Job drawing, mm, ordinate dimensions from the low corner. One solid piece. Round coordinates to 2 decimals unless told otherwise and drop trailing zeros. Loops run counter-clockwise (first coordinate to the right, second up) from the corner with the lowest first, then second, coordinate; pieces in that order, holes last.
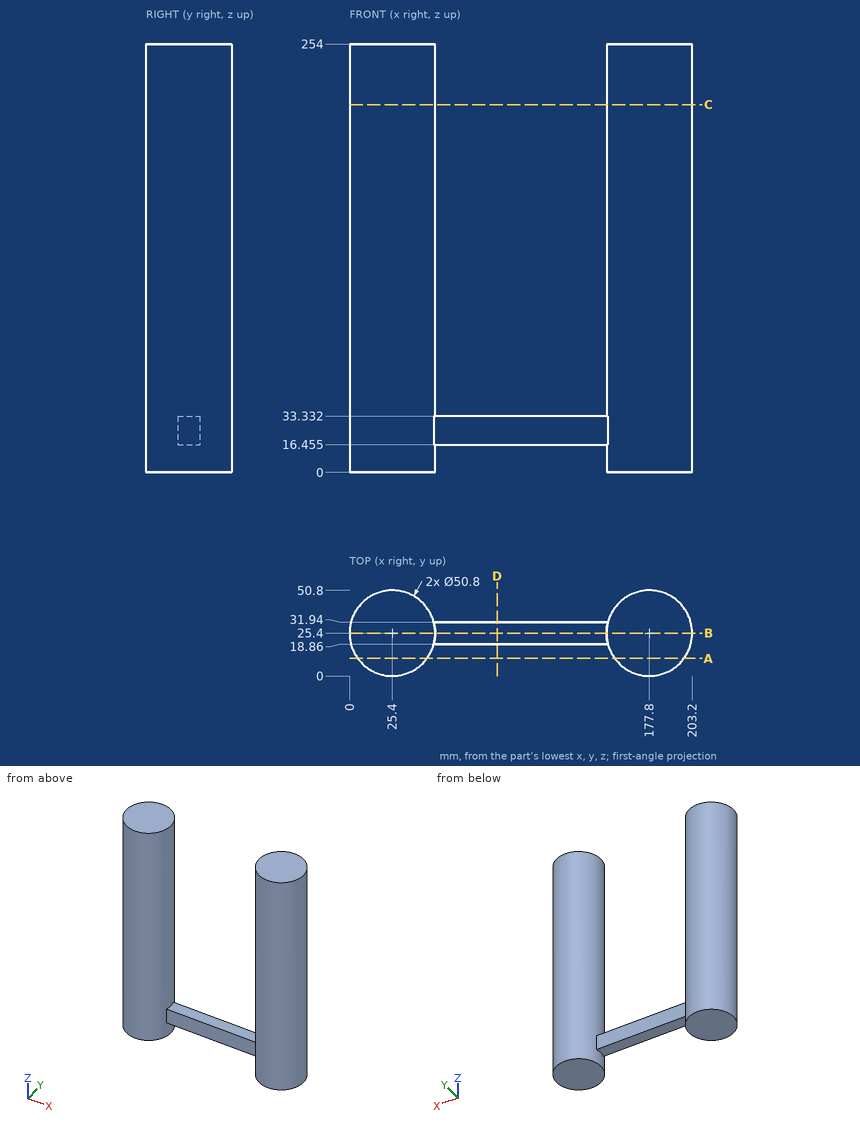
(1) Slice it at D-D on x = 87.5. List the corners of the cut face in (y, z) (1 decimal), plus the area to 3 significant figures.
Responses:
outline: (18.9, 16.5) - (31.9, 16.5) - (31.9, 33.3) - (18.9, 33.3) - close
area: 221 mm2
(2) Pin check, flat tips, straight feed: P1, Ø1.5, axis at y = 27, z = 194, coming from the -X side; P2, Ø8, axis at x = 111.5, y = 23, coming from the +Z side; P3, Ø3, axis at x = 155, z = 34.5, coming from the -Y side (1 decimal). Stop position of each tip, or through.
Responses:
P1: stops at x = 0.01
P2: stops at z = 33.33
P3: stops at y = 11.6
(3) Slice it at B-B on y = 25.4. List the corners of the cut face in (x, z) (1 decimal).
Responses:
outline: (0, 0) - (50.8, 0) - (50.8, 16.5) - (152.4, 16.5) - (152.4, 0) - (203.2, 0) - (203.2, 254) - (152.4, 254) - (152.4, 33.3) - (50.8, 33.3) - (50.8, 254) - (0, 254) - close
(4) Probe line 1 (Z direction, x = 104, y = 23.5) (1 decimal); line 2 (Y direction, x = 26.5, z = 17); line 3 (X direction, y = 8, z = 39.5) (1 decimal). List the from-to ranges inside material, lowest first.
Responses:
line 1: z = 16.5 to 33.3
line 2: y = 0.02 to 50.78
line 3: x = 6.9 to 43.9, 159.3 to 196.3
(5) Slice it at C-C on z = 218. List the corners of the cut face in (x, y).
Responses:
outline: circle Ø50.8 at (25.4, 25.4); circle Ø50.8 at (177.8, 25.4)
(6) Slice it at A-A on y = 10.5. List the corners of the cut face in (x, z).
Responses:
outline: (4.83, 0) - (45.97, 0) - (45.97, 254) - (4.83, 254) - close; (157.23, 0) - (198.37, 0) - (198.37, 254) - (157.23, 254) - close
